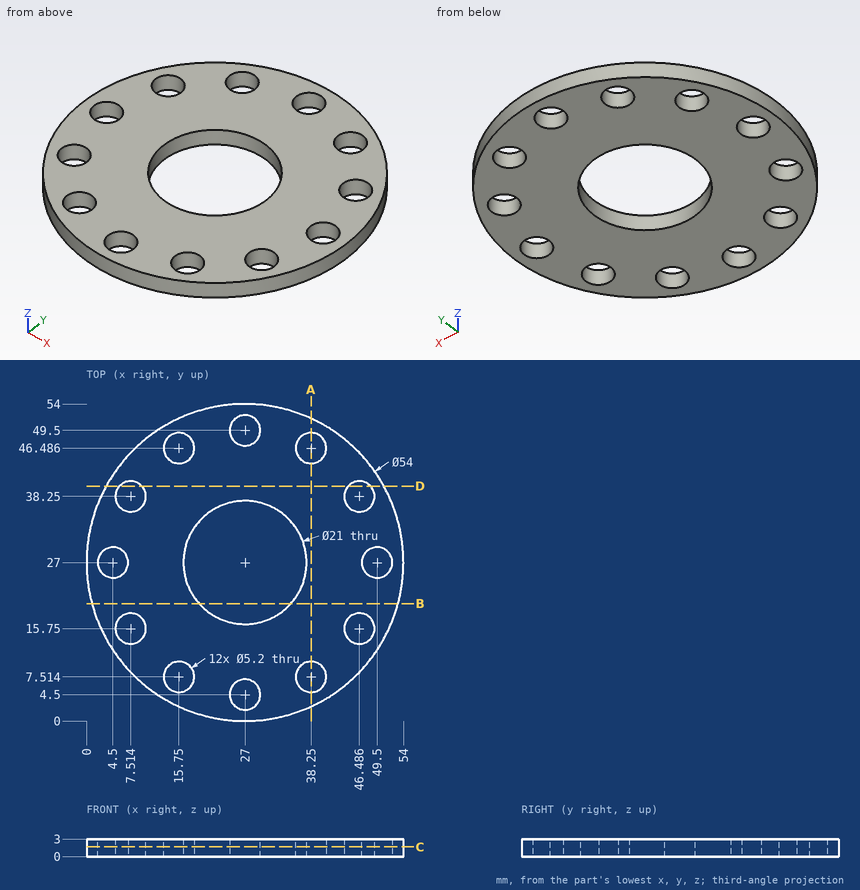
Study the drawing (mm; zero at the part's minimum x, y, z) and answer. Round coordinates to 2 decimals unless told otherwise and drop trailing zeros. Loops run counter-clockwise (first coordinate to the right, second up) from the corner with the lowest first, then second, coordinate; pieces in that order, holes last.
Q1. Given pin 1 Ø1 at (y, z) = (31, 1) entering from -X; pin 2 Ø1.5 at (x, z) = (40.5, 1) entering from -Y, each flat-ended and moving along its own axis, determine where each tip first touches the part or whether it passes through.
Q2. Section A-A, the plane x = 38.25 is taken. Determine the outline of the cut face in (y, z) (1 decimal), then the cut area to 3 significant figures.
Q3. Section D-D, the plane y = 40 is taken. Determine the outline of the cut face in (x, z) (1 decimal), then the cut area to 3 significant figures.
Q4. Find the intervals of material crossed by line 1 (X direction, y = 36.5, z = 2.1) (1 decimal); line 2 (Y direction, x = 38, z = 1.6) (1 decimal); line 3 (Y direction, x = 8, z = 2.75) (1 decimal), in increasing order.
Q5. Section B-B, the plane y = 20 is taken. Determine the outline of the cut face in (x, z).
Q6. Section C-C, the plane z = 1.65 is taken. Count the separate pieces of the cut face and the enclosed holes in it, then the cut area to 3 significant figures.
Completed:
1. pin 1: stops at x = 0.23
1. pin 2: stops at y = 3.2
2. outline: (2.5, 0) - (4.9, 0) - (4.9, 3) - (2.5, 3) - close; (10.1, 0) - (43.9, 0) - (43.9, 3) - (10.1, 3) - close; (49.1, 0) - (51.5, 0) - (51.5, 3) - (49.1, 3) - close
2. area: 116 mm2
3. outline: (3.3, 0) - (5.6, 0) - (5.6, 3) - (3.3, 3) - close; (9.4, 0) - (44.6, 0) - (44.6, 3) - (9.4, 3) - close; (48.4, 0) - (50.7, 0) - (50.7, 3) - (48.4, 3) - close
3. area: 119 mm2
4. line 1: x = 1.7 to 5.6, 9.4 to 22.5, 31.5 to 44.6, 48.4 to 52.3
4. line 2: y = 2.3 to 4.9, 10.1 to 43.9, 49.1 to 51.7
4. line 3: y = 7.8 to 13.2, 18.3 to 35.7, 40.8 to 46.2
5. outline: (0.92, 0) - (19.17, 0) - (19.17, 3) - (0.92, 3) - close; (34.83, 0) - (53.08, 0) - (53.08, 3) - (34.83, 3) - close
6. separate pieces: 1
6. enclosed holes: 13
6. area: 1,690 mm2
